from build123d import *

# Parameters (mm, degrees)
SKETCH1_R           = 2.1
BOSS_EXTRUDE1_DEPTH = 630


with BuildPart() as part:
    # Sketch1 → Boss-Extrude1 (new body)
    with BuildSketch(Plane(origin=(0, 0, 0), x_dir=(0, 0, -1), z_dir=(1, 0, 0))):
        with BuildLine():
            Line((-10, -13), (-10, -19))
            ThreePointArc((-10, -19), (-9.707106781, -19.707106781), (-9, -20))
            Line((-9, -20), (-3, -20))
            Line((-3, -20), (-3, -18))
            Line((-3, -18), (-6, -18))
            Line((-6, -18), (-6, -17.060660172))
            Line((-6, -17.060660172), (-2.939339828, -14))
            Line((-2.939339828, -14), (2.939339828, -14))
            Line((2.939339828, -14), (6, -17.060660172))
            Line((6, -17.060660172), (6, -18))
            Line((6, -18), (3, -18))
            Line((3, -18), (3, -20))
            Line((3, -20), (9, -20))
            ThreePointArc((9, -20), (9.707106781, -19.707106781), (10, -19))
            Line((10, -19), (10, -13))
            Line((10, -13), (8, -13))
            Line((8, -13), (8, -16))
            Line((8, -16), (7.060660172, -16))
            Line((7.060660172, -16), (4, -12.939339828))
            Line((4, -12.939339828), (4, -7.060660172))
            Line((4, -7.060660172), (7.060660172, -4))
            Line((7.060660172, -4), (8, -4))
            Line((8, -4), (8, -7))
            Line((8, -7), (10, -7))
            Line((10, -7), (10, 7))
            Line((10, 7), (8, 7))
            Line((8, 7), (8, 4))
            Line((8, 4), (7.060660172, 4))
            Line((7.060660172, 4), (4, 7.060660172))
            Line((4, 7.060660172), (4, 12.939339828))
            Line((4, 12.939339828), (7.060660172, 16))
            Line((7.060660172, 16), (8, 16))
            Line((8, 16), (8, 13))
            Line((8, 13), (10, 13))
            Line((10, 13), (10, 19))
            ThreePointArc((10, 19), (9.707106781, 19.707106781), (9, 20))
            Line((9, 20), (3, 20))
            Line((3, 20), (3, 18))
            Line((3, 18), (6, 18))
            Line((6, 18), (6, 17.060660172))
            Line((6, 17.060660172), (2.939339828, 14))
            Line((2.939339828, 14), (-2.939339828, 14))
            Line((-2.939339828, 14), (-6, 17.060660172))
            Line((-6, 17.060660172), (-6, 18))
            Line((-6, 18), (-3, 18))
            Line((-3, 18), (-3, 20))
            Line((-3, 20), (-9, 20))
            ThreePointArc((-9, 20), (-9.707106781, 19.707106781), (-10, 19))
            Line((-10, 19), (-10, 13))
            Line((-10, 13), (-8, 13))
            Line((-8, 13), (-8, 16))
            Line((-8, 16), (-7.060660172, 16))
            Line((-7.060660172, 16), (-4, 12.939339828))
            Line((-4, 12.939339828), (-4, 7.060660172))
            Line((-4, 7.060660172), (-7.060660172, 4))
            Line((-7.060660172, 4), (-8, 4))
            Line((-8, 4), (-8, 7))
            Line((-8, 7), (-10, 7))
            Line((-10, 7), (-10, -7))
            Line((-10, -7), (-8, -7))
            Line((-8, -7), (-8, -4))
            Line((-8, -4), (-7.060660172, -4))
            Line((-7.060660172, -4), (-4, -7.060660172))
            Line((-4, -7.060660172), (-4, -12.939339828))
            Line((-4, -12.939339828), (-7.060660172, -16))
            Line((-7.060660172, -16), (-8, -16))
            Line((-8, -16), (-8, -13))
            Line((-8, -13), (-10, -13))
        make_face()
        with Locations((0, 10)):
            Circle(SKETCH1_R, mode=Mode.SUBTRACT)
        with Locations((0, -10)):
            Circle(SKETCH1_R, mode=Mode.SUBTRACT)
        with BuildLine():
            Line((-8, 1.7), (-8, -1.7))
            ThreePointArc((-8, -1.7), (-7.912132034, -1.912132034), (-7.7, -2))
            Line((-7.7, -2), (-7.063603897, -2))
            ThreePointArc((-7.063603897, -2), (-6.948798867, -2.02283614), (-6.851471863, -2.087867966))
            Line((-6.851471863, -2.087867966), (-2.939339828, -6))
            Line((-2.939339828, -6), (2.939339828, -6))
            Line((2.939339828, -6), (6.851471863, -2.087867966))
            ThreePointArc((6.851471863, -2.087867966), (6.948798867, -2.02283614), (7.063603897, -2))
            Line((7.063603897, -2), (7.7, -2))
            ThreePointArc((7.7, -2), (7.912132034, -1.912132034), (8, -1.7))
            Line((8, -1.7), (8, 1.7))
            ThreePointArc((8, 1.7), (7.912132034, 1.912132034), (7.7, 2))
            Line((7.7, 2), (7.063603897, 2))
            ThreePointArc((7.063603897, 2), (6.948798867, 2.02283614), (6.851471863, 2.087867966))
            Line((6.851471863, 2.087867966), (2.939339828, 6))
            Line((2.939339828, 6), (-2.939339828, 6))
            Line((-2.939339828, 6), (-6.851471863, 2.087867966))
            ThreePointArc((-6.851471863, 2.087867966), (-6.948798867, 2.02283614), (-7.063603897, 2))
            Line((-7.063603897, 2), (-7.7, 2))
            ThreePointArc((-7.7, 2), (-7.912132034, 1.912132034), (-8, 1.7))
        make_face(mode=Mode.SUBTRACT)
    extrude(amount=BOSS_EXTRUDE1_DEPTH)


solid = part.part
Geometry: final body of the model. Coordinates: model frame, mm. Give positions to 0.01 mm unless a question says otherwise; leave off trailing zeros. Answer as a JSON object with one key per item and string values.
Q1. First-contact query: pin 1 (0.6 mm diameter, centred on x = 270, z = 9.5, fed in from +Y); pin 2 (3 mm diameter, centred on x = 436.5, y = -9, fed in from -Z); pin 3 (4 mm diameter, centred on x = 373, z = -0.5, fed in from -Y). Flat tips, straight axial feed; report the tip coordinate or a pass-through.
Entries:
{"pin 1": "stops at y = 19.98", "pin 2": "stops at z = -4", "pin 3": "stops at y = -14"}
Q2. Material intervals for probe 1 along Y at (x, z) = (411, 0); probe 2 along Y at (x, z) = (272, -8.75); probe 3 along Y at (x, z) = (574, 2.5), sorted ascending.
Entries:
{"probe 1": "y = -14 to -12.1, -7.9 to -6, 6 to 7.9, 12.1 to 14", "probe 2": "y = -20 to -13, -7 to 7, 13 to 20", "probe 3": "y = -14 to -6, 6 to 14"}
Q3. Section A-A (x = 385). State how many separate pieces and enclosed holes the cut face has, plus the area to 3 significant figures.
Entries:
{"separate pieces": "1", "enclosed holes": "3", "area": "325 mm^2"}
